Could you check a few things on this drawing? It's one solid part, dimensions in mm from its lowest x, y, z. Coordinates: 2 decimals unless noted, no trailing zeros. Loops run counter-clockwise (first coordinate to the right, second up) from the corner with the lowest first, then second, coordinate; pieces in that order, holes last.
1) Imagine slicing it at A-A on y = 1.27. Please give me the cut outline in (x, z) (3 decimals), plus the area to 3 significant figures.
2) Imagine slicing it at C-C on x = 1.27. Please give me the cut outline in (y, z) (3 decimals), plus the area to 3 significant figures.
3) Will this pin go through, and if not, where does the flat tip stop? P1, Ø1.3, axis at y = 1, z = 24.5, coming from the +X side.
4) Imagine slicing it at B-B on z = 15.5. Please give me the cut outline in (x, y).
5) If I drill on line 1 along Z through (x, y) = (1.25, 0.85) (3 decimals); line 2 along Y through (x, z) = (1.15, 12.5); line 3 along X through (y, z) = (1.35, 8), over which ranges is the centre line in solid material (lowest first)?
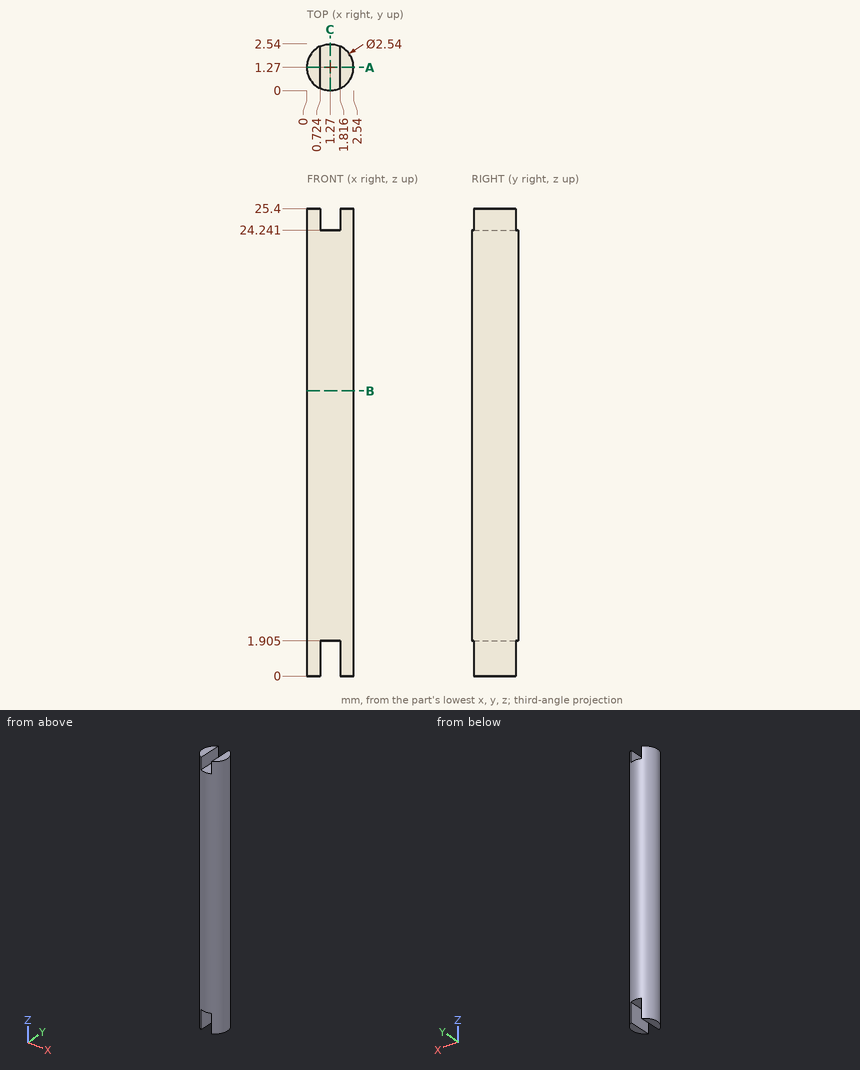
Filled in:
1. outline: (0, 0) - (0.724, 0) - (0.724, 1.905) - (1.816, 1.905) - (1.816, 0) - (2.54, 0) - (2.54, 25.4) - (1.816, 25.4) - (1.816, 24.241) - (0.724, 24.241) - (0.724, 25.4) - (0, 25.4) - close
1. area: 61.2 mm2
2. outline: (0, 1.905) - (2.54, 1.905) - (2.54, 24.241) - (0, 24.241) - close
2. area: 56.7 mm2
3. P1: stops at x = 2.54
4. outline: circle Ø2.54 at (1.27, 1.27)
5. line 1: z = 1.905 to 24.241
5. line 2: y = 0.01 to 2.53
5. line 3: x = 0 to 2.54
